Can you work these out from the model? Positions are in its coordinate system, mm. Face numbers are marked on the shaded views. A direction names the side the tool comes from. Round coordinates to 2 decimals unless told otherwise and drop trailing zeros. Loops run counter-clockwise (first coordinate to the right, second up) from the corner with the lowest first, then second, coordinate; pieces in that order, holes last. Notation, with made-up numbers: M 0,-12.75 L 51,-12.75 A30 cw 51,16.25 Z; hole C 43,6.5 d3. An arc over 180 degrees is marked long. Return JSON: item names as keys, results as strings.
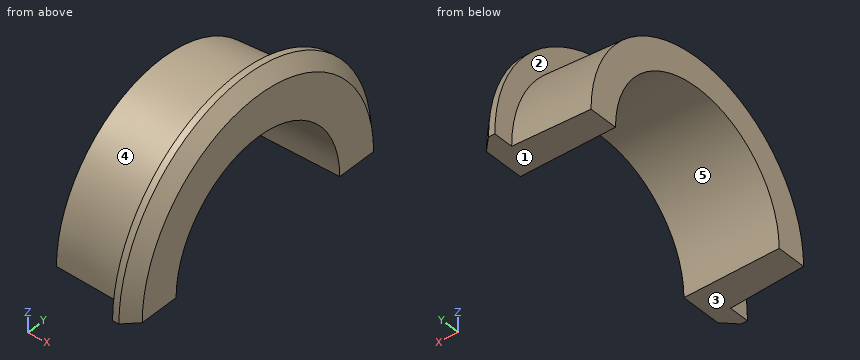
```python
from build123d import *

# Parameters (mm, degrees)
F2_ANGLE_BACK = 90
F2_ANGLE      = 180
F3_SIZE       = 2.54


with BuildPart() as f2:
    # F0 (on Front) → F2 (revolve)
    with BuildSketch(Plane.XZ, mode=Mode.PRIVATE) as f2_sk:
        Polygon((2.9366673195, 26.162), (-12.3033326805, 25.4), (-12.3033326805, 19.558), (6.7466673195, 19.558), (6.7466673195, 30.1889932623), (2.9366673195, 30.1889932623), align=None)
    revolve(f2_sk.sketch.rotate(Axis((-24.6385950595, 0, 0), (-1, 0, 0)), -F2_ANGLE_BACK), axis=Axis((-24.6385950595, 0, 0), (-1, 0, 0)), revolution_arc=F2_ANGLE)

    # F3
    f3_edges = [f2.edges().sort_by_distance(p)[0] for p in [
        (6.746667, 0, 30.188993),
    ]]
    chamfer(f3_edges, length=F3_SIZE)


solid = f2.part
```
Q1. Suppose I cut it at C-C, the plane x = -5. Please give me the cut outline in (y, z).
Results:
{"outline": "M -25.77,0 L -19.56,0 A19.56 cw 19.56,0 L 25.77,0 A25.77 ccw Z"}
Q2. Suppose I cut it at B-B, the plane x = 3.5. Please give me the cut outline in (y, z), plus the area to 3 significant figures.
Results:
{"outline": "M -30.19,0 L -19.56,0 A19.56 cw 19.56,0 L 30.19,0 A30.19 ccw Z", "area": "831 mm2"}
Q3. If I drill on line 1 along X through (y, z) = (21, 17); line 2 along Y through (x, z) = (0.5, 10); line 3 along Y through (x, z) = (0.25, 3), over which ranges is the centre line in solid material (lowest first)?
Results:
{"line 1": "x = 2.94 to 6.75", "line 2": "y = -24.04 to -16.81, 16.81 to 24.04", "line 3": "y = -25.85 to -19.33, 19.33 to 25.85"}
Q4. Suppose I cut it at A-A, the plane y = 0. Please give me the cut outline in (x, z), plus the area to 3 significant figures.
Results:
{"outline": "M -12.3,19.56 L 6.75,19.56 L 6.75,27.65 L 4.21,30.19 L 2.94,30.19 L 2.94,26.16 L -12.3,25.4 Z", "area": "132 mm2"}
Q5. I'm going to push flat-ended pins straight in: pin 1 Ø5 at (x, z) = (3.5, 5) entering from -Y; pin 2 Ø1 at (x, z) = (-8, 18) entering from -Y; pin 3 Ø2 at (x, z) = (-4.5, 24.5) entering from -Y. Where does each tip first touch, or does it pass through?
Results:
{"pin 1": "stops at y = -30.09", "pin 2": "stops at y = -18.71", "pin 3": "stops at y = -10.63"}
Q6. On a 3-axis mill with a long thin cutter (end or side, diameter ignored), from which of +Z, -Z, +X, -X, +Y, -Y can I reach the whole of each face in a straight line? I mean the marked faces 1 and 2. Say none if no direction works.
Results:
{"face 1": "-Z, +X, -X, +Y, -Y", "face 2": "+Z, -X"}
Q7. Thinking about a two-plate mould opening in Y: for the marked faces 3, 4 and 5, which applies, pulls with the +Y half, pulls with the -Y half, needs draft (parallel to the pull), parting line crosses it, or undercut?
Results:
{"face 3": "needs draft", "face 4": "parting line crosses it", "face 5": "undercut"}
